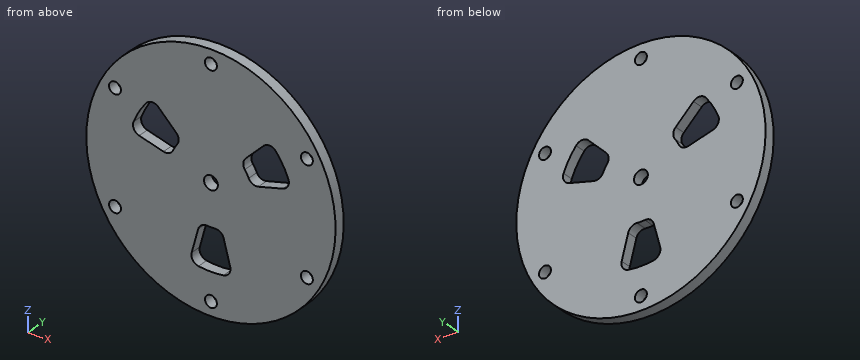
```python
from build123d import *

# Parameters (mm, degrees)
SKETCH_1_R      = 45
SKETCH_1_R_2    = 2.15
SKETCH_1_R_3    = 2.5
EXTRUDE_1_DEPTH = 2


with BuildPart() as part:
    # Эскиз1 → Бобышка-Вытянуть1 (new, symmetric)
    with BuildSketch(Plane(origin=(0, 0, 0), x_dir=(1, 0, 0), z_dir=(0, 1, 0))):
        with Locations(Location((0, 0, 0), (0, 0, 270))):
            Circle(SKETCH_1_R)
        with Locations(Location((0, 40, 0), (0, 0, 270))):
            Circle(SKETCH_1_R_2, mode=Mode.SUBTRACT)
        with Locations(Location((0, -40, 0), (0, 0, 90))):
            Circle(SKETCH_1_R_2, mode=Mode.SUBTRACT)
        with Locations(Location((34.641016151, -20, 0), (0, 0, 270))):
            Circle(SKETCH_1_R_2, mode=Mode.SUBTRACT)
        with Locations(Location((-34.641016151, 20, 0), (0, 0, 90))):
            Circle(SKETCH_1_R_2, mode=Mode.SUBTRACT)
        with Locations(Location((-34.641016151, -20, 0), (0, 0, 270))):
            Circle(SKETCH_1_R_2, mode=Mode.SUBTRACT)
        with Locations(Location((34.641016151, 20, 0), (0, 0, 90))):
            Circle(SKETCH_1_R_2, mode=Mode.SUBTRACT)
        with Locations(Location((0, 0, 0), (0, 0, 270))):
            Circle(SKETCH_1_R_3, mode=Mode.SUBTRACT)
        with BuildLine():
            Line((-6.944843745, 25.918509706), (-4.593582361, 17.143482759))
            ThreePointArc((-4.593582361, 17.143482759), (-3.407818063, 15.456403642), (-1.413170735, 14.933283245))
            ThreePointArc((-1.413170735, 14.933283245), (0, 15), (1.413170735, 14.933283245))
            ThreePointArc((1.413170735, 14.933283245), (3.407818063, 15.456403642), (4.593582361, 17.143482759))
            Line((4.593582361, 17.143482759), (6.944843745, 25.918509706))
            ThreePointArc((6.944843745, 25.918509706), (6.557654897, 28.33720456), (4.496740295, 29.661074268))
            ThreePointArc((4.496740295, 29.661074268), (0, 30), (-4.496740295, 29.661074268))
            ThreePointArc((-4.496740295, 29.661074268), (-6.557654897, 28.33720456), (-6.944843745, 25.918509706))
        make_face(mode=Mode.SUBTRACT)
        with BuildLine():
            Line((18.973665961, -18.973665961), (12.549900398, -12.549900398))
            ThreePointArc((12.549900398, -12.549900398), (11.681729173, -10.679458835), (12.226017285, -8.690483379))
            ThreePointArc((12.226017285, -8.690483379), (12.990381057, -7.5), (13.639188019, -6.242799866))
            ThreePointArc((13.639188019, -6.242799866), (15.089547237, -4.776944806), (17.143482759, -4.593582361))
            Line((17.143482759, -4.593582361), (25.918509706, -6.944843745))
            ThreePointArc((25.918509706, -6.944843745), (27.819566469, -8.48950655), (27.935613967, -10.936245804))
            ThreePointArc((27.935613967, -10.936245804), (25.980762114, -15), (23.438873672, -18.724828464))
            ThreePointArc((23.438873672, -18.724828464), (21.261911572, -19.84769801), (18.973665961, -18.973665961))
        make_face(mode=Mode.SUBTRACT)
        with BuildLine():
            Line((-25.918509706, -6.944843745), (-17.143482759, -4.593582361))
            ThreePointArc((-17.143482759, -4.593582361), (-15.089547237, -4.776944806), (-13.639188019, -6.242799866))
            ThreePointArc((-13.639188019, -6.242799866), (-12.990381057, -7.5), (-12.226017285, -8.690483379))
            ThreePointArc((-12.226017285, -8.690483379), (-11.681729173, -10.679458835), (-12.549900398, -12.549900398))
            Line((-12.549900398, -12.549900398), (-18.973665961, -18.973665961))
            ThreePointArc((-18.973665961, -18.973665961), (-21.261911572, -19.84769801), (-23.438873672, -18.724828464))
            ThreePointArc((-23.438873672, -18.724828464), (-25.980762114, -15), (-27.935613967, -10.936245804))
            ThreePointArc((-27.935613967, -10.936245804), (-27.819566469, -8.48950655), (-25.918509706, -6.944843745))
        make_face(mode=Mode.SUBTRACT)
    extrude(amount=EXTRUDE_1_DEPTH, both=True)


solid = part.part
```
Work out the finished part from the listing and answer in its coordinate system (mm). Give positions to 0.01 mm unless a question says otherwise; leave off trailing zeros. Write each loop counter-clockwise with the first axis right and the second up, starting at its lowest first coordinate (ties: lowest second). Pieces come first, ordered by that corner, then holes.
(1) The part is cut by section B-B on x = 0. Write down the section's boundary in (y, z).
Final values:
outline: (-2, -45) - (2, -45) - (2, -42.15) - (-2, -42.15) - close; (-2, -37.85) - (2, -37.85) - (2, -30) - (-2, -30) - close; (-2, -15) - (2, -15) - (2, -2.5) - (-2, -2.5) - close; (-2, 2.5) - (2, 2.5) - (2, 37.85) - (-2, 37.85) - close; (-2, 42.15) - (2, 42.15) - (2, 45) - (-2, 45) - close
(2) The part is cut by section D-D on y = -0.45. Count the separate pieces of the cut face and the enclosed holes in it, plus the area to 3 significant figures.
Final values:
separate pieces: 1
enclosed holes: 10
area: 5,750 mm2
(3) The part is cut by section C-C on z = -20. Write down the section's boundary in (x, y).
Final values:
outline: (-40.31, -2) - (-36.79, -2) - (-36.79, 2) - (-40.31, 2) - close; (-32.49, -2) - (-5.36, -2) - (-5.36, 2) - (-32.49, 2) - close; (5.36, -2) - (32.49, -2) - (32.49, 2) - (5.36, 2) - close; (36.79, -2) - (40.31, -2) - (40.31, 2) - (36.79, 2) - close
(4) Straight lines are drawn through the part: line 1 (X direction, y = -1.5, z = -18.5); line 2 (X direction, y = 0.2, z = 20); line 3 (X direction, y = -1.05, z = 9). For each, find the intervals that lie inside material, in ascending order.
Final values:
line 1: x = -41.02 to -36.18, -33.1 to -4.96, 4.96 to 33.1, 36.18 to 41.02
line 2: x = -40.31 to -36.79, -32.49 to 32.49, 36.79 to 40.31
line 3: x = -44.09 to -28.02, -12.03 to 12.03, 28.02 to 44.09
(5) The part is cut by section A-A on z = 0. Write down the section's boundary in (x, y).
Final values:
outline: (-45, -2) - (-2.5, -2) - (-2.5, 2) - (-45, 2) - close; (2.5, -2) - (45, -2) - (45, 2) - (2.5, 2) - close
(6) Flat-ended cylindrical pins translate along their axes: pin 1 Ø4 at (x, z) = (0, 0) entering from +Y; pin 2 Ø1 at (x, y) = (-22, 0) entering from +Z; pin 3 Ø2 at (y, z) = (-1.5, -1.5) entering from -X; pin 4 Ø2 at (y, z) = (1.5, 1) entering from +X. Find the tip coordinate at first contact, or state that the pin passes through.
Final values:
pin 1: passes through
pin 2: stops at z = 39.53
pin 3: stops at x = -45
pin 4: stops at x = 45
